Build history of the part. All positions in model axes, mm. A direction names the side the tool comes from. Give positions to 0.01 mm unless a question says otherwise; leave off trailing zeros. Loops run counter-clockwise (first coordinate to the right, second up) from the corner with the lowest first, then second, coordinate; pieces in that order, holes last. Notation, with made-up numbers: (42.25, 30.25) -> (63.25, 30.25) arc R16 cw to (63.25, 37.25) -> close; hole circle Ø8 at (47.5, 64.25). An arc over 180 degrees is marked (long way). Answer as a JSON object with one key per item and string values. Group by question number.
Q1. Drop flat-ended pins along their axis: pin 1 (4.5 mm diameter, centred on y = 7.5, z = 4.5, fed in from +X); pin 2 (4.5 mm diameter, centred on y = -12, z = 2.5, fed in from -X); pin 3 (4.5 mm diameter, centred on y = -6.5, z = 3, fed in from +X). Give the stop position or say it passes through.
Q2. Band-saw the part on A-A, the plane y = 7. Write the cut outline in (x, z), plus the area to 3 significant figures.
Q3. Two-plate mould, pull along X, no slides. Class faces 4 (the flat face through (27, -23, 4)), 5 (the flat face through (32.27, -18.94, 4.44)), 6 (the flat face through (38, 5, 4)), 7 (the flat face through (24.77, -19.06, 4.44)): pulls with the +X half, pulls with the -X half, needs draft (parallel to the pull), parting line crosses it, or undercut.
Q4. Band-saw the part on D-D, the plane y = -1. Write the cut outline in (x, z), plus the area to 3 significant figures.
Q5. Tool access for faces 1 (the flat face through (33, -15, 4)), 2 (the flat face through (35, 6, 4)), 3 (the flat face through (57, 8, 4)): list every direction of +Z, -Z, +X, -X, +Y, -Y with a clear straight run to the whole face (end or side of a thin tool).
Q6. Band-saw the part on B-B, the plane y = -6. Write the cut outline in (x, z), plus the area to 3 significant figures.
Q7. Band-saw the part on C-C, the plane z = 3. Write the cut outline in (x, y), plus the area to 3 significant figures.
Q8. Wall check: probe 1 along X at (y, z) = (8, 4.25); probe 2 along X at (y, z) = (-10, 1.25); probe 3 along X at (y, z) = (17.5, 7). Give the ranges that are in metal, low to high. Write a range as from..to.
from build123d import *

# Parameters (mm, degrees)
BOSS_EXTRUDE1_DEPTH = 9


with BuildPart() as part:
    # Sketch1 → Boss-Extrude1 (new body)
    with BuildSketch(Plane.XY):
        with BuildLine():
            Line((0, 3), (0, 12))
            ThreePointArc((0, 12), (11, 23), (22, 12))
            Line((22, 12), (22, 0))
            Line((22, 0), (35, 0))
            Line((35, 0), (35, 12))
            ThreePointArc((35, 12), (46, 23), (57, 12))
            Line((57, 12), (57, 3))
            ThreePointArc((57, 3), (59.121320344, -2.121320344), (54, 0))
            Line((54, 0), (54, 12))
            ThreePointArc((54, 12), (46, 20), (38, 12))
            Line((38, 12), (38, -3))
            Line((38, -3), (32, -3))
            Line((32, -3), (32, -15))
            Line((32, -15), (33.5, -15))
            Line((33.5, -15), (31, -23))
            Line((31, -23), (29.5, -23))
            Line((29.5, -23), (29.5, -3))
            ThreePointArc((29.5, -3), (28.5, -2), (27.5, -3))
            Line((27.5, -3), (27.5, -23))
            Line((27.5, -23), (26, -23))
            Line((26, -23), (23.5, -15))
            Line((23.5, -15), (25, -15))
            Line((25, -15), (25, -3))
            Line((25, -3), (19, -3))
            Line((19, -3), (19, 12))
            ThreePointArc((19, 12), (11, 20), (3, 12))
            Line((3, 12), (3, 0))
            ThreePointArc((3, 0), (-2.121320344, -2.121320344), (0, 3))
        make_face()
    extrude(amount=BOSS_EXTRUDE1_DEPTH)


solid = part.part
Worked answers:
{
 "1": {"pin 1": "x = 57", "pin 2": "x = 25", "pin 3": "x = 32"},
 "2": {"outline": "(0, 0) -> (3, 0) -> (3, 9) -> (0, 9) -> close; (19, 0) -> (22, 0) -> (22, 9) -> (19, 9) -> close; (35, 0) -> (38, 0) -> (38, 9) -> (35, 9) -> close; (54, 0) -> (57, 0) -> (57, 9) -> (54, 9) -> close", "area": "108 mm2"},
 "3": {"face 4": "needs draft", "face 5": "pulls with the +X half", "face 6": "undercut", "face 7": "pulls with the -X half"},
 "4": {"outline": "(-2.83, 0) -> (2.83, 0) -> (2.83, 9) -> (-2.83, 9) -> close; (19, 0) -> (38, 0) -> (38, 9) -> (19, 9) -> close; (54.17, 0) -> (59.83, 0) -> (59.83, 9) -> (54.17, 9) -> close", "area": "273 mm2"},
 "5": {"face 1": "+Z, -Z, +X", "face 2": "+Z, -Z, +Y", "face 3": "+Z, -Z, +X, +Y"},
 "6": {"outline": "(25, 0) -> (27.5, 0) -> (27.5, 9) -> (25, 9) -> close; (29.5, 0) -> (32, 0) -> (32, 9) -> (29.5, 9) -> close", "area": "45.0 mm2"},
 "7": {"outline": "(0, 3) arc R3 ccw (long way) to (3, 0) -> (3, 12) arc R8 cw to (19, 12) -> (19, -3) -> (25, -3) -> (25, -15) -> (23.5, -15) -> (26, -23) -> (27.5, -23) -> (27.5, -3) arc R1 cw to (29.5, -3) -> (29.5, -23) -> (31, -23) -> (33.5, -15) -> (32, -15) -> (32, -3) -> (38, -3) -> (38, 12) arc R8 cw to (54, 12) -> (54, 0) arc R3 ccw (long way) to (57, 3) -> (57, 12) arc R11 ccw to (35, 12) -> (35, 0) -> (22, 0) -> (22, 12) arc R11 ccw to (0, 12) -> close", "area": "525 mm2"},
 "8": {"probe 1": "0..3, 19..22, 35..38, 54..57", "probe 2": "25..27.5, 29.5..32", "probe 3": "1.47..5.19, 16.81..20.53, 36.47..40.19, 51.81..55.53"}
}
